CAD build for the part. Positions are in the model's coordinates, mm. A direction names the side the tool comes from. Coordinates: 2 decimals unless noted, no trailing zeros. Order: outer loops, then holes, each group sorted by start corner. A loop starts at its lowest first (then second) coordinate and runs counter-clockwise, first axis right, second up.
from build123d import *

# Parameters (mm, degrees)
BOSS_EXTRUDE2_DEPTH     = 69.5
BOSS_EXTRUDE3_DEPTH     = 69.5
CUT_EXTRUDE1_DEPTH      = 77.467274154
CUT_EXTRUDE1_DEPTH_BACK = 77.467274154
SKETCH7_R               = 2
CUT_EXTRUDE2_DEPTH      = 78.205129928
CUT_EXTRUDE2_DEPTH_BACK = 78.205129928
SKETCH8_R               = 1.7


with BuildPart() as part:
    # Sketch4 → Boss-Extrude2 (new body)
    with BuildSketch(Plane.XY):
        Polygon((-4.302602112, 10.373468411), (-10.302602112, 10.373468411), (-10.302602112, -5.626531589), (-4.302602112, -5.626531589), (-4.302602112, -2.286531589), (-5.712602112, -2.286531589), (-6.832602112, -3.406531589), (-7.462602112, -3.406531589), (-7.462602112, 8.153468411), (-6.832602112, 8.153468411), (-5.712602112, 7.033468411), (-4.302602112, 7.033468411), align=None)
    extrude(amount=BOSS_EXTRUDE2_DEPTH)

    # Sketch6 → Boss-Extrude3 (add)
    with BuildSketch(Plane.XY.offset(69.5)):
        with BuildLine():
            Line((-18.82375255, 27.373468411), (-23.82375255, 27.373468411))
            Line((-23.82375255, 27.373468411), (-23.82375255, 15.03032266))
            ThreePointArc((-23.82375255, 15.03032266), (-23.51927068, 13.499588931), (-22.652179675, 12.201895535))
            Line((-22.652179675, 12.201895535), (-20.82375255, 10.373468411))
            Line((-20.82375255, 10.373468411), (-20.82375255, -5.626531589))
            Line((-20.82375255, -5.626531589), (-22.652179675, -7.454958714))
            ThreePointArc((-22.652179675, -7.454958714), (-23.51927068, -8.752652109), (-23.82375255, -10.283385839))
            Line((-23.82375255, -10.283385839), (-23.82375255, -22.626531589))
            Line((-23.82375255, -22.626531589), (-18.82375255, -22.626531589))
            Line((-18.82375255, -22.626531589), (-18.82375255, -11.458931103))
            ThreePointArc((-18.82375255, -11.458931103), (-18.088209901, -9.14736925), (-16.152093449, -7.685933561))
            Line((-16.152093449, -7.685933561), (-10.302602112, -5.626531589))
            Line((-10.302602112, -5.626531589), (-10.302602112, 10.373468411))
            Line((-10.302602112, 10.373468411), (-16.820008224, 12.668019889))
            ThreePointArc((-16.820008224, 12.668019889), (-18.272095564, 13.764096656), (-18.82375255, 15.497768046))
            Line((-18.82375255, 15.497768046), (-18.82375255, 27.373468411))
        make_face()
    extrude(amount=-BOSS_EXTRUDE3_DEPTH)

    # Sketch7 → Cut-Extrude1 (cut, two sides: drawn at the far end of the back side and taken through both)
    with BuildSketch(Plane(origin=(-7.462602112, 0, 0), x_dir=(0, 0, -1), z_dir=(1, 0, 0)).offset(-CUT_EXTRUDE1_DEPTH_BACK)):
        with Locations(Location((-34.5, 2.373468411, 0), (0, 0, 180))):
            Circle(SKETCH7_R)
        with Locations(Location((-14.5, 2.373468411, 0), (0, 0, 180))):
            Circle(SKETCH7_R)
    extrude(amount=CUT_EXTRUDE1_DEPTH + CUT_EXTRUDE1_DEPTH_BACK, mode=Mode.SUBTRACT)

    # Sketch8 → Cut-Extrude2 (cut, two sides: drawn at the far end of the back side and taken through both)
    with BuildSketch(Plane.ZY.offset(23.82375255).offset(-CUT_EXTRUDE2_DEPTH_BACK)):
        with Locations(Location((12, 19.373468411, 0), (0, 0, 270))):
            Circle(SKETCH8_R)
        with Locations(Location((57.5, 19.373468411, 0), (0, 0, 270))):
            Circle(SKETCH8_R)
        with Locations(Location((57.5, -14.626531589, 0), (0, 0, 270))):
            Circle(SKETCH8_R)
        with Locations(Location((12, -14.626531589, 0), (0, 0, 270))):
            Circle(SKETCH8_R)
    extrude(amount=CUT_EXTRUDE2_DEPTH + CUT_EXTRUDE2_DEPTH_BACK, mode=Mode.SUBTRACT)


solid = part.part
1) Two-plate mould, pull along Z, no slides. Class faces 5 (the cylindrical face through (-21, -16, 13)), 6 (the flat face through (-4.303, 9, 34)), 7 (the flat face through (-16, 3, 69.5)): released by +Z, released by -Z, zero draft, split by the parting line, or undercut.
2) Drill centre lines: probe 1 along X at (y, z) = (-13, 5.5); probe 2 along Y at (x, z) = (-7.25, 16.5); probe 3 along X at (y, z) = (3.5, 31). Where is each one in solid material? Low to high.
3) Slice it at C-C (z = 24). List the corners of the cut face in (x, y).
4) Slice it at B-B (z = 57.5). Give the number of separate pieces and of enclosed holes in the cut face, plus the area to 3 significant figures.
5) Which spindle directions (+Z, -Z, +X, -X, +Y, -Y) get a long thin tool onto all of the face, cutting with end or side? Do faces 1 (the flat face through (-18.824, 21, 35)), 2 (the flat face through (-5, -2.287, 34)), 3 (the cylindrical face through (-23.528, 13.52, 35.236)), 4 (the flat face through (-18.824, -17, 35)). Say none if no direction does.
6) Slice it at D-D (x = -15). List the corners of the cut face in (y, z).
7) Pin check, flat tips, straight feed: P1, Ø6, axis at y = -15, z = 48, coming from the +X side; P2, Ø0.7, axis at x = -7, z = 50.5, coming from the -Y side; P3, Ø5, axis at y = 2.37, z = 14.5, coming from the -X side. Stop position of each tip, or through.
Worked out:
1. face 5: undercut
1. face 6: zero draft
1. face 7: released by +Z
2. probe 1: x = -23.82 to -18.82
2. probe 2: y = -5.63 to -3.41, 8.15 to 10.37
2. probe 3: x = -20.82 to -7.46
3. outline: (-23.82, -22.63) - (-18.82, -22.63) - (-18.82, -11.46) arc R4 cw to (-16.15, -7.69) - (-10.3, -5.63) - (-4.3, -5.63) - (-4.3, -2.29) - (-5.71, -2.29) - (-6.83, -3.41) - (-7.46, -3.41) - (-7.46, 8.15) - (-6.83, 8.15) - (-5.71, 7.03) - (-4.3, 7.03) - (-4.3, 10.37) - (-10.3, 10.37) - (-16.82, 12.67) arc R3 cw to (-18.82, 15.5) - (-18.82, 27.37) - (-23.82, 27.37) - (-23.82, 15.03) arc R4 ccw to (-22.65, 12.2) - (-20.82, 10.37) - (-20.82, -5.63) - (-22.65, -7.45) arc R4 ccw to (-23.82, -10.28) - close
4. separate pieces: 3
4. enclosed holes: 0
4. area: 386 mm2
5. face 1: +Z, -Z, +X, +Y
5. face 2: +Z, -Z, +X
5. face 3: +Z, -Z, -X
5. face 4: +Z, -Z, +X, -Y
6. outline: (-7.28, 0) - (12.03, 0) - (12.03, 69.5) - (-7.28, 69.5) - close; hole circle Ø4 at (2.37, 14.5); hole circle Ø4 at (2.37, 34.5)
7. P1: stops at x = -18.82
7. P2: stops at y = -5.63
7. P3: stops at x = -20.82
